Job drawing, mm, ordinate dimensions from the low corner. One solid piece. Give positions to 0.01 mm unless a question says otherwise; leave off trailing zeros. Loops run counter-clockwise (first coordinate to the right, second up) from the corner with the lowest first, then second, coordinate; pieces in that order, holes last. Notation, with made-up numbers: M -20,-13 L -9,-13 A12 ccw -9,-5 Z; hole C 80,7.5 d7. An arc over 180 degrees is marked long. Answer as CSV lines item,"result".
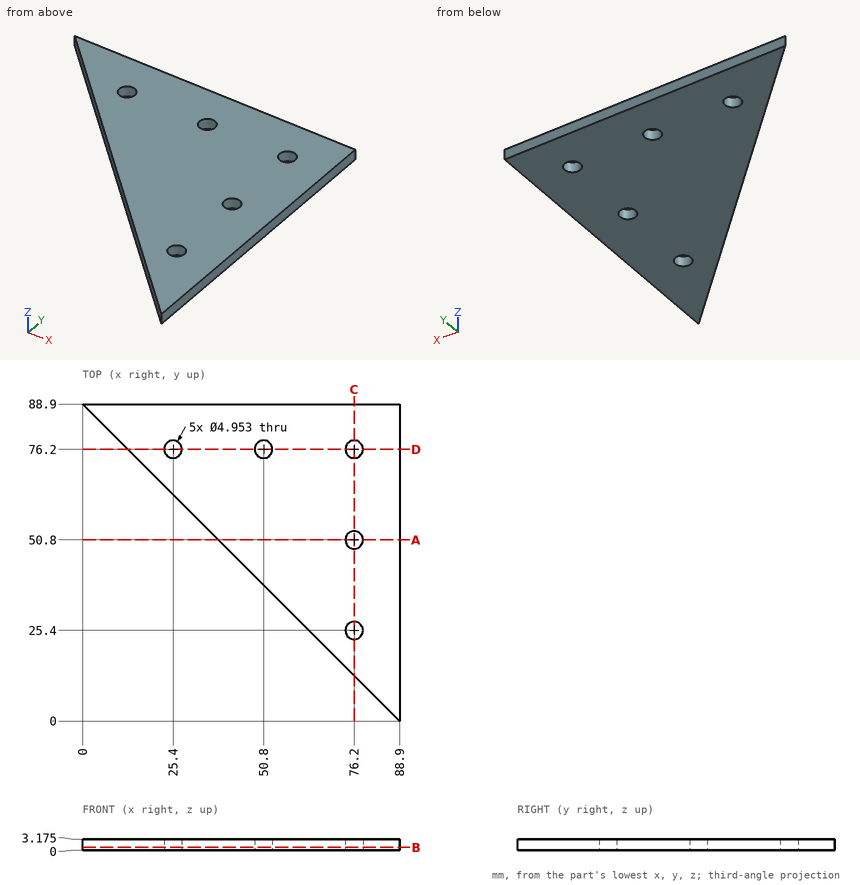
1) Flat gauge pin, fed straight in: pin 1 (12 mm diameter, centred on x = 18.5, y = 66, fed in from -Z). Where does the tip first touch, or does it go through?
Answer below:
pin 1,"stops at z = 0"
2) Band-saw the part on C-C on x = 76.2. Give the cut face in (y, z) (1 decimal).
Answer below:
outline,"M 12.7,0 L 22.9,0 L 22.9,3.2 L 12.7,3.2 Z; M 27.9,0 L 48.3,0 L 48.3,3.2 L 27.9,3.2 Z; M 53.3,0 L 73.7,0 L 73.7,3.2 L 53.3,3.2 Z; M 78.7,0 L 88.9,0 L 88.9,3.2 L 78.7,3.2 Z"
3) Band-saw the part on B-B on z = 0.8. Give the cut face in (x, y).
Answer below:
outline,"M 0,88.9 L 88.9,0 L 88.9,88.9 Z; hole C 25.4,76.2 d4.95; hole C 50.8,76.2 d4.95; hole C 76.2,25.4 d4.95; hole C 76.2,50.8 d4.95; hole C 76.2,76.2 d4.95"
4) Drill centre lines: line 1 (Y direction, x = 76.2, z = 1.3); line 2 (Y direction, x = 77.5, z = 0.2); line 3 (Y direction, x = 6, z = 1.85). Where is each one in solid material? Low to high. Write a range as from..to.
Answer below:
line 1,"y = 12.7..22.92, 27.88..48.32, 53.28..73.72, 78.68..88.9"
line 2,"y = 11.4..23.29, 27.51..48.69, 52.91..74.09, 78.31..88.9"
line 3,"y = 82.9..88.9"
5) Band-saw the part on A-A on y = 50.8. Give the cut face in (x, z) (1 decimal).
Answer below:
outline,"M 38.1,0 L 73.7,0 L 73.7,3.2 L 38.1,3.2 Z; M 78.7,0 L 88.9,0 L 88.9,3.2 L 78.7,3.2 Z"
